Here's how the part is built. I have some questions about the finished solid (model axes, mm). A direction names the side the tool comes from. Round coordinates to 2 decimals unless told otherwise and drop trailing zeros. Loops run counter-clockwise (first coordinate to the right, second up) from the corner with the lowest first, then second, coordinate; pieces in that order, holes last. Notation, with made-up numbers: M 44.5,73 L 97.5,73 A28 ccw 97.5,97 Z; hole C 72,17.5 d1. An arc over 180 degrees is marked long. Answer as a JSON object with one key per item and string values.
from build123d import *

# Parameters (mm, degrees)
SKETCH1_W           = 37.465
SKETCH1_H           = 24.13
BOSS_EXTRUDE1_DEPTH = 4.445
CUT_EXTRUDE2_DEPTH  = 2.54
FILLET1_R           = 5.08
CUT_EXTRUDE4_DEPTH  = 2.54
SKETCH4_R           = 1.27
CUT_EXTRUDE5_DEPTH  = 2.54
SKETCH5_R           = 1.905
SKETCH5_R_2         = 1.27
CUT_EXTRUDE6_DEPTH  = 0.635
CUT_EXTRUDE7_DEPTH  = 2.54
BOSS_EXTRUDE2_START = 2.54
SKETCH7_R           = 1.905
BOSS_EXTRUDE2_DEPTH = 2.54
SKETCH8_R           = 1
CUT_EXTRUDE8_DEPTH  = 45.784385114


with BuildPart() as part:
    # Sketch1 → Boss-Extrude1 (new body)
    with BuildSketch(Plane.XY):
        with Locations((18.7325, 12.065)):
            Rectangle(SKETCH1_W, SKETCH1_H)
    extrude(amount=BOSS_EXTRUDE1_DEPTH)

    # Sketch2 → Cut-Extrude2 (cut)
    # profile 1 of 4: a face of its own
    with BuildSketch(Plane.XY.offset(4.445)):
        with BuildLine():
            Line((35.59175, 5.7785), (35.59175, 12.065))
            Line((35.59175, 12.065), (35.59175, 18.3515))
            ThreePointArc((35.59175, 18.3515), (34.135361545, 21.710109865), (30.681521372, 22.9235))
            Line((30.681521372, 22.9235), (18.7325, 22.9235))
            Line((18.7325, 22.9235), (6.107021372, 22.9235))
            ThreePointArc((6.107021372, 22.9235), (3.090639267, 21.470453234), (1.87325, 18.3515))
            Line((1.87325, 18.3515), (1.87325, 12.065))
            Line((1.87325, 12.065), (1.87325, 5.7785))
            ThreePointArc((1.87325, 5.7785), (3.212357796, 2.545607796), (6.44525, 1.2065))
            Line((6.44525, 1.2065), (18.7325, 1.2065))
            Line((18.7325, 1.2065), (31.01975, 1.2065))
            ThreePointArc((31.01975, 1.2065), (34.252642204, 2.545607796), (35.59175, 5.7785))
        make_face()
        with BuildLine():
            ThreePointArc((7.493, 3.175), (4.439712919, 4.439712919), (3.175, 7.493))
            Line((3.175, 7.493), (3.175, 16.637))
            ThreePointArc((3.175, 16.637), (4.317872951, 19.576666289), (7.154771372, 20.955))
            Line((7.154771372, 20.955), (7.493, 20.955))
            Line((7.493, 20.955), (29.633771372, 20.955))
            ThreePointArc((29.633771372, 20.955), (32.908147923, 19.81638289), (34.29, 16.637))
            Line((34.29, 16.637), (34.29, 7.493))
            ThreePointArc((34.29, 7.493), (33.025287081, 4.439712919), (29.972, 3.175))
            Line((29.972, 3.175), (7.493, 3.175))
        make_face(mode=Mode.SUBTRACT)
    # profile 2 of 4: a face of its own
    with BuildSketch(Plane.XY.offset(4.445)):
        with BuildLine():
            ThreePointArc((3.175, 16.637), (4.439712919, 19.690287081), (7.493, 20.955))
            Line((7.493, 20.955), (29.972, 20.955))
            ThreePointArc((29.972, 20.955), (33.025287081, 19.690287081), (34.29, 16.637))
            Line((34.29, 16.637), (34.29, 7.493))
            ThreePointArc((34.29, 7.493), (33.025287081, 4.439712919), (29.972, 3.175))
            Line((29.972, 3.175), (7.493, 3.175))
            ThreePointArc((7.493, 3.175), (4.439712919, 4.439712919), (3.175, 7.493))
            Line((3.175, 7.493), (3.175, 16.637))
        make_face()
    # profile 3 of 4: a face of its own
    with BuildSketch(Plane.XY.offset(4.445)):
        with BuildLine():
            ThreePointArc((7.154771372, 20.955), (4.317872951, 19.576666289), (3.175, 16.637))
            ThreePointArc((3.175, 16.637), (4.439712919, 19.690287081), (7.493, 20.955))
            Line((7.493, 20.955), (7.154771372, 20.955))
        make_face()
    # profile 4 of 4: a face of its own
    with BuildSketch(Plane.XY.offset(4.445)):
        with BuildLine():
            ThreePointArc((34.29, 16.637), (32.908147923, 19.81638289), (29.633771372, 20.955))
            Line((29.633771372, 20.955), (29.972, 20.955))
            ThreePointArc((29.972, 20.955), (33.025287081, 19.690287081), (34.29, 16.637))
        make_face()
    extrude(amount=-CUT_EXTRUDE2_DEPTH, mode=Mode.SUBTRACT)

    # Fillet1
    fillet1_edges = [part.edges().sort_by_distance(p)[0] for p in [
        (0, 24.13, 2.2225),
        (37.465, 24.13, 2.2225),
        (37.465, 0, 2.2225),
        (0, 0, 2.2225),
    ]]
    fillet(fillet1_edges, radius=FILLET1_R)

    # Sketch3 → Cut-Extrude4 (cut)
    with BuildSketch(Plane.XY.offset(1.905)):
        with BuildLine():
            Line((7.350869654, 16.158973759), (18.677995313, 16.158973759))
            ThreePointArc((18.677995313, 16.158973759), (21.522821275, 14.644991178), (22.463869654, 11.5628481))
            Line((22.463869654, 11.5628481), (22.463869654, 7.801099417))
            ThreePointArc((22.463869654, 7.801099417), (21.522821275, 4.718956339), (18.677995313, 3.204973759))
            Line((18.677995313, 3.204973759), (7.350869654, 3.204973759))
            ThreePointArc((7.350869654, 3.204973759), (4.387385134, 4.432489239), (3.159869654, 7.395973759))
            Line((3.159869654, 7.395973759), (3.159869654, 11.967973759))
            ThreePointArc((3.159869654, 11.967973759), (4.387385134, 14.931458278), (7.350869654, 16.158973759))
        make_face()
    extrude(amount=-CUT_EXTRUDE4_DEPTH, mode=Mode.SUBTRACT)

    # Sketch4 → Cut-Extrude5 (cut)
    with BuildSketch(Plane.XY.offset(1.905)):
        with Locations((27.511650569, 9.68988988)):
            Circle(SKETCH4_R)
    extrude(amount=-CUT_EXTRUDE5_DEPTH, mode=Mode.SUBTRACT)

    # Sketch5 → Cut-Extrude6 (cut)
    with BuildSketch(Plane.XY.offset(1.905)):
        with Locations((27.511650569, 9.68988988)):
            Circle(SKETCH5_R)
        with Locations((27.511650569, 9.68988988)):
            Circle(SKETCH5_R_2, mode=Mode.SUBTRACT)
    extrude(amount=-CUT_EXTRUDE6_DEPTH, mode=Mode.SUBTRACT)

    # Sketch6 → Cut-Extrude7 (cut)
    with BuildSketch(Plane.XY.offset(4.445)):
        with BuildLine():
            Line((1.542829573, 18.47723), (1.542829573, 5.65277))
            ThreePointArc((1.542829573, 5.65277), (2.908719525, 2.355219952), (6.206269573, 0.98933))
            Line((6.206269573, 0.98933), (31.272259573, 0.98933))
            ThreePointArc((31.272259573, 0.98933), (34.56980962, 2.355219952), (35.935699573, 5.65277))
            Line((35.935699573, 5.65277), (35.935699573, 18.47723))
            ThreePointArc((35.935699573, 18.47723), (34.450183348, 21.903012063), (30.927266372, 23.14067))
            Line((30.927266372, 23.14067), (5.861276372, 23.14067))
            ThreePointArc((5.861276372, 23.14067), (2.784566625, 21.658562299), (1.542829573, 18.47723))
        make_face()
        with BuildLine():
            Line((6.44525, 1.2065), (31.01975, 1.2065))
            ThreePointArc((31.01975, 1.2065), (34.252642204, 2.545607796), (35.59175, 5.7785))
            Line((35.59175, 5.7785), (35.59175, 18.3515))
            ThreePointArc((35.59175, 18.3515), (34.135361545, 21.710109865), (30.681521372, 22.9235))
            Line((30.681521372, 22.9235), (6.107021372, 22.9235))
            ThreePointArc((6.107021372, 22.9235), (3.090639267, 21.470453234), (1.87325, 18.3515))
            Line((1.87325, 18.3515), (1.87325, 5.7785))
            ThreePointArc((1.87325, 5.7785), (3.212357796, 2.545607796), (6.44525, 1.2065))
        make_face(mode=Mode.SUBTRACT)
    extrude(amount=-CUT_EXTRUDE7_DEPTH, mode=Mode.SUBTRACT)

    # Sketch7 → Boss-Extrude2 (add)
    with BuildSketch(Plane.XY.offset(1.905).offset(BOSS_EXTRUDE2_START)):
        with BuildLine():
            Line((1.542829573, 18.47723), (1.542829573, 5.65277))
            ThreePointArc((1.542829573, 5.65277), (2.908719525, 2.355219952), (6.206269573, 0.98933))
            Line((6.206269573, 0.98933), (31.272259573, 0.98933))
            ThreePointArc((31.272259573, 0.98933), (34.56980962, 2.355219952), (35.935699573, 5.65277))
            Line((35.935699573, 5.65277), (35.935699573, 18.47723))
            ThreePointArc((35.935699573, 18.47723), (34.450183348, 21.903012063), (30.927266372, 23.14067))
            Line((30.927266372, 23.14067), (5.861276372, 23.14067))
            ThreePointArc((5.861276372, 23.14067), (2.784566625, 21.658562299), (1.542829573, 18.47723))
        make_face()
        with Locations((27.511650569, 9.68988988)):
            Circle(SKETCH7_R, mode=Mode.SUBTRACT)
        with BuildLine():
            Line((3.159869654, 7.395973759), (3.159869654, 11.967973759))
            ThreePointArc((3.159869654, 11.967973759), (4.387385134, 14.931458278), (7.350869654, 16.158973759))
            Line((7.350869654, 16.158973759), (18.677995313, 16.158973759))
            ThreePointArc((18.677995313, 16.158973759), (21.522821275, 14.644991178), (22.463869654, 11.5628481))
            Line((22.463869654, 11.5628481), (22.463869654, 7.801099417))
            ThreePointArc((22.463869654, 7.801099417), (21.522821275, 4.718956339), (18.677995313, 3.204973759))
            Line((18.677995313, 3.204973759), (7.350869654, 3.204973759))
            ThreePointArc((7.350869654, 3.204973759), (4.387385134, 4.432489239), (3.159869654, 7.395973759))
        make_face(mode=Mode.SUBTRACT)
    extrude(amount=-BOSS_EXTRUDE2_DEPTH)

    # Sketch8 → Cut-Extrude8 (cut, through all)
    with BuildSketch(Plane(origin=(0, 0, 0), x_dir=(-1, 0, 0), z_dir=(0, 0, -1))):
        with Locations((-34.499249276, 21.164249276)):
            Circle(SKETCH8_R)
        with Locations((-34.499249276, 2.965750724)):
            Circle(SKETCH8_R)
        with Locations((-2.965750724, 2.965750724)):
            Circle(SKETCH8_R)
        with Locations((-2.965750724, 21.164249276)):
            Circle(SKETCH8_R)
    extrude(amount=-CUT_EXTRUDE8_DEPTH, mode=Mode.SUBTRACT)


solid = part.part
Item 1: For faces 1 (the face through (21.493, 14.681, 2.254)), 2 (the face through (37.465, 12, 2)), 3 (the face through (29.27, 8.96, 2.88)), which set-ups out of +Z, -Z, +X, -X, +Y, -Y let a thin tool reach every point of the face, with its end or its side?
Solution:
{"face 1": "+Z, -Z", "face 2": "+Z, -Z, +X, +Y, -Y", "face 3": "+Z"}
Item 2: I want a section at A-A on x = 13.5. List the corners of the cut face in (y, z) for me (3 decimals), plus the area to 3 significant figures.
Solution:
{"outline": "M 0,0 L 3.205,0 L 3.205,4.445 L 0,4.445 Z; M 16.159,0 L 24.13,0 L 24.13,4.445 L 16.159,4.445 Z", "area": "49.7 mm2"}
Item 3: If I drill on L1, parallel to X at y = 11, z = 0.45 (3 decimals); L2, parallel to Y at x = 35, z = 1.5; L3, parallel to Y at x = 13, z = 2, over which ranges is the centre line in solid material (lowest first)? Write a range as from..to.
Solution:
{"L1": "x = 0..3.16, 22.464..37.465", "L2": "y = 0.72..2.1, 3.83..20.3, 22.03..23.41", "L3": "y = 0..3.2, 16.16..24.13"}
Item 4: We'd pull the mould along Y, two halves only. Please class faces 4 (the face through (4.42, 4.4, 2.25)), 5 (the face through (1.449, 1.528, 2.254)), 6 (the face through (22.464, 10, 2)), 7 (the face through (23, 12, 4.445)): +Y half, -Y half, draft (parallel to the pull), parting line (faces both ways), or undercut.
Solution:
{"face 4": "undercut", "face 5": "-Y half", "face 6": "undercut", "face 7": "draft"}
Item 5: I want a section at D-D on y = 9.25. List the corners of the cut face in (x, z) for me (3 decimals).
Solution:
{"outline": "M 0,0 L 3.16,0 L 3.16,4.445 L 0,4.445 Z; M 22.464,0 L 26.32,0 L 26.32,1.27 L 25.658,1.27 L 25.658,4.445 L 22.464,4.445 Z; M 28.703,0 L 37.465,0 L 37.465,4.445 L 29.365,4.445 L 29.365,1.27 L 28.703,1.27 Z"}
Item 6: I want a section at B-B on y = 6.25. List the corners of the cut face in (x, z) for me (3 decimals).
Solution:
{"outline": "M 0,0 L 3.32,0 L 3.32,4.445 L 0,4.445 Z; M 22.324,0 L 37.465,0 L 37.465,4.445 L 22.324,4.445 Z"}
Item 7: I want a section at C-C on z = 1.75. List the corners of the cut face in (x, y) for me (3 decimals), plus the area to 3 significant figures.
Solution:
{"outline": "M 0,5.08 A5.08 ccw 5.08,0 L 32.385,0 A5.08 ccw 37.465,5.08 L 37.465,19.05 A5.08 ccw 32.385,24.13 L 5.08,24.13 A5.08 ccw 0,19.05 Z; hole C 2.966,2.966 d2; hole C 2.966,21.164 d2; hole M 3.16,7.396 A4.191 ccw 7.351,3.205 L 18.678,3.205 A4.211 ccw 22.464,7.801 L 22.464,11.563 A4.211 ccw 18.678,16.159 L 7.351,16.159 A4.191 ccw 3.16,11.968 Z; hole C 27.512,9.69 d3.81; hole C 34.499,2.966 d2; hole C 34.499,21.164 d2", "area": "623 mm2"}
